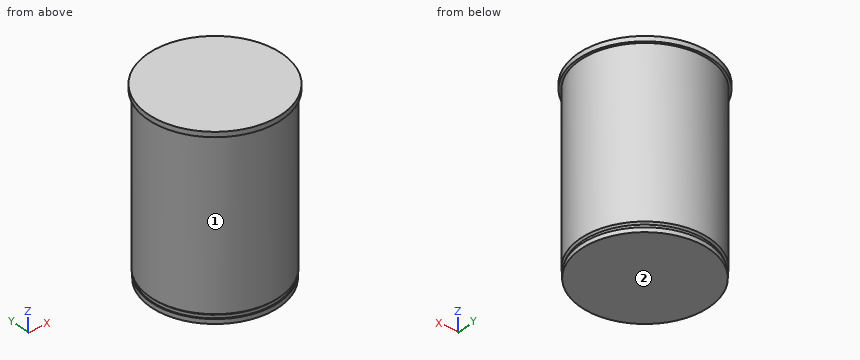
from build123d import *

# Parameters (mm, degrees)
F0_R        = 35.8775
F1_DEPTH    = 2.54
F2_R        = 35.21075
F3_DEPTH    = 1.778
F4_R        = 36.195
F5_DEPTH    = 93.853
F6_R        = 37.465
F7_DEPTH    = 2.794
F8_S5_R     = 35.21075
F8_T6_DEPTH = 53


# Not quite as in the source:
# - a fillet or chamfer that OpenCascade refuses, or shapes differently, is made with other operations: its cross-section is extruded or revolved along the edge and cut away or added


with BuildPart() as f1:
    # F0 (on Top) → F1 (new body)
    with BuildSketch(Plane.XY):
        Circle(F0_R)
    extrude(amount=F1_DEPTH)

    # F2 (on face) → F3 (join)
    with BuildSketch(Plane.XY.offset(2.54)):
        Circle(F2_R)
    extrude(amount=F3_DEPTH)

    # F4 (on face) → F5 (join)
    with BuildSketch(Plane.XY.offset(4.318)):
        Circle(F4_R)
    extrude(amount=F5_DEPTH)

    # F6 (on face) → F7 (join)
    with BuildSketch(Plane.XY.offset(98.171)):
        Circle(F6_R)
    extrude(amount=F7_DEPTH)

    # F8: chamfer of 1.016 on 1 edges, made by hand


with BuildPart() as f8_tool2:
    # F8_s3 → F8_t4 (revolve)
    with BuildSketch(Plane.XZ):
        Polygon((36.195, 5.334), (35.179, 4.318), (36.195, 4.318), align=None)
    revolve(axis=Axis((0, 0, 4.318), (0, 0, 1)))

    # F8_s5 → F8_t6 (cut, symmetric)
    with BuildSketch(Plane.XY.offset(4.8)):
        Circle(F8_S5_R)
    extrude(amount=F8_T6_DEPTH, both=True, mode=Mode.SUBTRACT)


with BuildPart() as f1_1:
    add(f1.part)

    # F8_t1: cut F8_tool2
    add(f8_tool2.part, mode=Mode.SUBTRACT)


solid = f1_1.part
Check sheet for the modelled part. Datum: model origin and axes. Units: mm. Face numbers are marked on the shaded views. A direction names the side the tool comes from. Give positions to 0.01 mm unless a question says otherwise; leave off trailing zeros. Order: outer loops, then holes, each group sorted by start corner. A loop starts at its lowest first (then second) coordinate and runs counter-clockwise, first axis right, second up. Notation, with made-up numbers: (35.25, -20) - (47.25, -20) arc R17 cw to (47.25, 2) - close; hole circle Ø5 at (-32, 38.25). An arc over 180 degrees is marked (long way). Answer as CSV lines item,"result".
1. Tool access check on the marked faces 1 and 2. Record the directions out of +Z, -Z, +X, -X, +Y, -Y that give a thin tool (end or side, any length) a straight path to the whole face; none if there is none.
Result sheet:
face 1,"-Z"
face 2,"-Z, +X, -X, +Y, -Y"
2. Go/stop test with flat-tipped pins: P1, Ø12, axis at x = 29, z = 30.5, coming from the +Y side; P2, Ø8, axis at x = 7, z = 13.5, coming from the -Y side; P3, Ø8, axis at y = 9, z = 19.5, coming from the -X side. Record where each tip stops, or that it passes through.
Result sheet:
P1,"y = 27.95"
P2,"y = -36.07"
P3,"x = -35.85"
3. Section check C-C (z = 23.5). Record the boundary of the cut face in (x, y) (3 decimals), then the cut area to 3 significant figures.
Result sheet:
outline,"circle Ø72.39 at (0, 0)"
area,"4,120 mm²"
4. Section check A-A (y = 0). Record the boundary of the cut face in (x, z) (1 decimal).
Result sheet:
outline,"(-37.5, 98.2) - (-36.2, 98.2) - (-36.2, 5.3) - (-35.2, 4.3) - (-35.2, 2.5) - (-35.9, 2.5) - (-35.9, 0) - (35.9, 0) - (35.9, 2.5) - (35.2, 2.5) - (35.2, 4.3) - (36.2, 5.3) - (36.2, 98.2) - (37.5, 98.2) - (37.5, 101) - (-37.5, 101) - close"
5. Scan lines: probe 1 along Y at (x, z) = (-1, 90); probe 2 along Y at (x, z) = (-12.5, 9); probe 3 along X at (y, z) = (26, 63). Record each from-to range of solid material in increasing order. Write a range as from..to.
Result sheet:
probe 1,"-36.18..36.18"
probe 2,"-33.97..33.97"
probe 3,"-25.18..25.18"
